Autodesk Fusion 360 part; units mm, degrees
sketch "Sketch1" plane through (0, 0, 0) normal (0, 0, 1) x (1, 0, 0)
  circle A0 centre (0, 0) radius 30
  circle A1 centre (129, 0) radius 20
  line L0 (129, 15) -> (114.7342, 4.6353)
  line L1 (114.7342, 4.6353) -> (120.1832, -12.1353)
  line L2 (120.1832, -12.1353) -> (137.8168, -12.1353)
  line L3 (137.8168, -12.1353) -> (143.2658, 4.6353)
  line L4 (143.2658, 4.6353) -> (129, 15)
  line L5 (-11.547, 20) -> (-23.094, 0)
  line L6 (-23.094, 0) -> (-11.547, -20)
  line L7 (-11.547, -20) -> (11.547, -20)
  line L8 (11.547, -20) -> (23.094, 0)
  line L9 (23.094, 0) -> (11.547, 20)
  line L10 (11.547, 20) -> (-11.547, 20)
  line L11 (28.2843, 10) -> (111.6795, 10)
  line L12 (28.2843, -10) -> (111.6795, -10)
  line L13 (100, 5) -> (40, 5)
  line L14 (40, -5) -> (100, -5)
  line L15 (105, 5) -> (35, -5) construction
  line L16 (35, 5) -> (105, -5) construction
  arc A2 (40, 5) -> (40, -5) centre (40, 0) ccw
  arc A3 (100, -5) -> (100, 5) centre (100, 0) ccw
  point P0 (129, 0)
  point P1 (70, 0)
  dimension "d6" = 129
  dimension "d9" = 20
  dimension "d10" = 60
  dimension "d11" = 40
  dimension "d12" = 15
  dimension "d17" = 70
  dimension "d18" = 10
extrude "Extrude1" add sketch "Sketch1" along normal mid plane 20 contours A0 | A1 makes body 1 at (27.1662, -12.7278, 3.3333) makes body 2 at (148.9006, -1.9914, -3.3333)
extrude "Extrude2" add sketch "Sketch1" along normal mid plane 12 contours A0 A1 L11 L12 bodies 1 2
extrude "Extrude3" add sketch "Sketch1" along normal blind 3 contours L13 L14 A2 A3 bodies 1
Input: part model. Units: mm. Frame: model coordinates. A direction names the side the tool comes from. Round coordinates to 2 decimals unless told otherwise and drop trailing zeros. Loops run counter-clockwise (first coordinate to the right, second up) from the corner with the lowest first, then second, coordinate; pieces in that order, holes last. Notation, with made-up numbers: M 18,-26 L 32,-26 A18 cw 32,4 Z; hole C 36.25,10.25 d8. An arc over 180 degrees is marked long. Answer in a Markdown table with one row per item. Add a question column.
1. Section B-B (z = -4). Output: boundary loops of the cut face in (x, y).
2. Section C-C (y = -17.5). Output: boundary loops of the cut face in (x, z), and give its area (3 significant figures).
3. Section D-D (x = 21). Output: boundary loops of the cut face in (y, z), and give its area (3 significant figures).
4. Contact query for flat-ended pins moving along their axis: pin 1 (9 mm diameter, centred on x = 129, z = -1, fed in from +Y); pin 2 (3.5 mm diameter, centred on x = 49, z = 0, fed in from +Y); pin 3 (5 mm diameter, centred on x = -2, z = 1.5, fed in from -Y). Output: stop coordinate, or through.
5. Mould query, pull axis Y, two halves, no side actions, for faces 1 (the face through (-29.97, -1.32, -0.14)), 2 (the face through (20, 7, 10)), 3 (the face through (0, 20, 0)). Classes: released by +Y, released by -Y, zero draft, split by the parting line, or undercut.
6. Section A-A (x = 70). Output: boundary loops of the cut face in (y, z).
7. Set-up query: faces 4 (the face through (69, -10, 0)), 5 (the face through (70, 5, -3)), 6 (the face through (70, 0, 3)), 7 (the face through (117.42, -3.63, -0.14)), 8 (the face through (69, 10, 0)). Return all of +Z, -Z, +X, -X, +Y, -Y with unobstructed straight access to the full face (end or side cutting, diameter ignored); none if empty.
8. Ray query, probe 1 along Y at (x, z) = (44, 4.25); probe 2 along X at (y, z) = (-13.5, -0.75); probe 3 along Y at (x, z) = (84.5, 1.25). Return the intervals inside material, ascending.
Values follow:
| question | item | result |
|---|---|---|
| 1 | outline | M 28.28,-10 L 111.68,-10 A20 ccw long 111.68,10 L 28.28,10 A30 ccw long Z; hole M -23.09,0 L -11.55,-20 L 11.55,-20 L 23.09,0 L 11.55,20 L -11.55,20 Z; hole M 40,-5 L 100,-5 A5 ccw 100,5 L 40,5 A5 ccw Z; hole M 114.73,4.64 L 120.18,-12.14 L 137.82,-12.14 L 143.27,4.64 L 129,15 Z |
| 2 | outline | M -24.37,-10 L -12.99,-10 L -12.99,10 L -24.37,10 Z; M 12.99,-10 L 24.37,-10 L 24.37,10 L 12.99,10 Z; M 119.32,-10 L 138.68,-10 L 138.68,10 L 119.32,10 Z |
| 2 | area | 842 mm^2 |
| 3 | outline | M -21.42,-10 L -3.63,-10 L -3.63,10 L -21.42,10 Z; M 3.63,-10 L 21.42,-10 L 21.42,10 L 3.63,10 Z |
| 3 | area | 712 mm^2 |
| 4 | pin 1 | y = 20 |
| 4 | pin 2 | y = 10 |
| 4 | pin 3 | y = -30 |
| 5 | face 1 | split by the parting line |
| 5 | face 2 | zero draft |
| 5 | face 3 | undercut |
| 6 | outline | M -10,-6 L -5,-6 L -5,0 L 5,0 L 5,-6 L 10,-6 L 10,6 L 5,6 L 5,3 L -5,3 L -5,6 L -10,6 Z |
| 7 | face 4 | +Z, -Z, -Y |
| 7 | face 5 | -Z |
| 7 | face 6 | +Z |
| 7 | face 7 | +Z, -Z |
| 7 | face 8 | +Z, -Z, +Y |
| 8 | probe 1 | -10 to -5, 5 to 10 |
| 8 | probe 2 | -26.79 to -15.3, 15.3 to 26.79, 114.24 to 143.76 |
| 8 | probe 3 | -10 to 10 |
